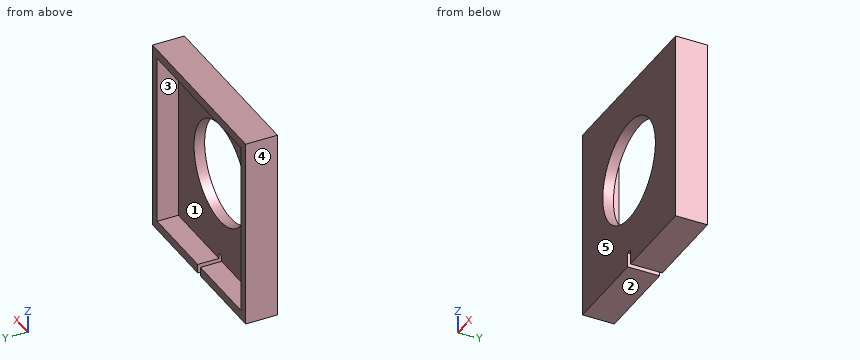
```python
from build123d import *

# Parameters (mm, degrees)
SKETCH1_W           = 34
SKETCH1_H           = 36
BOSS_EXTRUDE1_DEPTH = 6
SKETCH2_W           = 30.6
SKETCH2_H           = 32.6
CUT_EXTRUDE1_DEPTH  = 4
SKETCH3_R           = 9.6
CUT_EXTRUDE2_DEPTH  = 50.879855653
SKETCH4_W           = 1
SKETCH4_H           = 2.8
CUT_EXTRUDE3_DEPTH  = 50.879855653


with BuildPart() as part:
    # Sketch1 → Boss-Extrude1 (new body)
    with BuildSketch(Plane(origin=(0, 0, 0), x_dir=(1, 0, 0), z_dir=(0, 1, 0))):
        with Locations((17, 18)):
            Rectangle(SKETCH1_W, SKETCH1_H)
    extrude(amount=BOSS_EXTRUDE1_DEPTH)

    # Sketch2 → Cut-Extrude1 (cut)
    with BuildSketch(Plane(origin=(0, 6, 0), x_dir=(1, 0, 0), z_dir=(0, 1, 0))):
        with Locations((17, 18)):
            Rectangle(SKETCH2_W, SKETCH2_H)
    extrude(amount=-CUT_EXTRUDE1_DEPTH, mode=Mode.SUBTRACT)

    # Sketch3 → Cut-Extrude2 (cut, through all)
    with BuildSketch(Plane.XZ):
        with Locations(Location((17, -17, 0), (0, 0, 270))):
            Circle(SKETCH3_R)
    extrude(amount=-CUT_EXTRUDE2_DEPTH, mode=Mode.SUBTRACT)

    # Sketch4 → Cut-Extrude3 (cut, through all)
    with BuildSketch(Plane.XZ):
        with Locations((17, -34.6)):
            Rectangle(SKETCH4_W, SKETCH4_H)
    extrude(amount=-CUT_EXTRUDE3_DEPTH, mode=Mode.SUBTRACT)


solid = part.part
```
Geometry check sheet. Reference: the model listing, model coordinates, mm. Face numbers are marked on the shaded views. A direction names the side the tool comes from. Give positions to 0.01 mm unless a question says otherwise; leave off trailing zeros. Loops run counter-clockwise (first coordinate to the right, second up) from the corner with the lowest first, then second, coordinate; pieces in that order, holes last. Notation, with made-up numbers: M 44.25,3 L 74.25,3 A22 cw 74.25,35 Z; hole C 1,-27.5 d2. An arc over 180 degrees is marked long. Write item = value, one per line. Start each with the question number.
1. Draft check along X on the marked faces 3, 4 and 5. Enter one of: +X half, -X half, draft (parallel to the pull), parting line (faces both ways), or undercut.
2. Section check B-B, the plane z = -17. Enter the section's corners in (x, y).
3. Thickness scan on probe 1 along X at (y, z) = (0.5, -17); probe 2 along X at (y, z) = (2.5, -17.5); probe 3 along Z at (x, y) = (8.5, 5.75). Record the ranges inside material, lowest first.
4. Tool access check on the marked faces 1 and 2. Record the directions out of +Z, -Z, +X, -X, +Y, -Y that give a thin tool (end or side, any length) a straight path to the whole face; none if there is none.
5. Section check C-C, the plane z = -27. Enter the section's corners in (x, y), plus the area to 3 significant figures.
6. Go/stop test with flat-tipped pins: P1, Ø10, axis at x = 13.5, z = -10.5, coming from the -Y side; P2, Ø9, axis at x = 10.5, z = -23.5, coming from the +Y side. Record where each tip stops, or that it passes through.
7. Section check D-D, the plane y = 4.6. Enter the section's corners in (x, z), plus the area to 3 significant figures.
8. Section check A-A, the plane x = 17. Enter the section's corners in (y, z), plus the area to 3 significant figures.
Values follow:
q1.face_3 = undercut
q1.face_4 = -X half
q1.face_5 = draft
q2.outline = M 0,0 L 7.4,0 L 7.4,2 L 1.7,2 L 1.7,6 L 0,6 Z; M 26.6,0 L 34,0 L 34,6 L 32.3,6 L 32.3,2 L 26.6,2 Z
q3.probe_1 = 0 to 7.4, 26.6 to 34
q3.probe_2 = 0 to 1.7, 32.3 to 34
q3.probe_3 = -36 to -34.3, -1.7 to 0
q4.face_1 = +Y
q4.face_2 = -Z, +X, -X, +Y, -Y
q5.outline = M 0,0 L 34,0 L 34,6 L 32.3,6 L 32.3,2 L 1.7,2 L 1.7,6 L 0,6 Z
q5.area = 81.6 mm^2
q6.P1 = 0
q6.P2 = 2
q7.outline = M 0,-36 L 16.5,-36 L 16.5,-34.3 L 1.7,-34.3 L 1.7,-1.7 L 32.3,-1.7 L 32.3,-34.3 L 17.5,-34.3 L 17.5,-36 L 34,-36 L 34,0 L 0,0 Z
q7.area = 225 mm^2
q8.outline = M 0,-33.2 L 2,-33.2 L 2,-26.6 L 0,-26.6 Z; M 0,-7.4 L 2,-7.4 L 2,-1.7 L 6,-1.7 L 6,0 L 0,0 Z
q8.area = 34.8 mm^2
